Source: CAD feature listing. Evaluate the final solid. Frame: model axes, mm. A direction names the side the tool comes from. Round coordinates to 2 decimals unless told otherwise and drop trailing zeros. Loops run counter-clockwise (first coordinate to the right, second up) from the corner with the lowest first, then second, coordinate; pieces in that order, holes last. Notation, with made-up numbers: (71.5, -36) - (84.5, -36) arc R29 cw to (84.5, -1) - close; hole circle Ø4 at (-8, -39.75). An arc over 180 degrees is marked (long way). Write item = value, one per line. Start each with the question number.
from build123d import *

# Parameters (mm, degrees)
SKETCH1_R           = 5
BOSS_EXTRUDE1_DEPTH = 50
FILLET2_R           = 10
SKETCH2_R           = 12.5
CUT_EXTRUDE2_DEPTH  = 10


with BuildPart() as part:
    # Sketch1 → Boss-Extrude1 (new body)
    with BuildSketch(Plane.XY):
        with BuildLine():
            Line((0, 0), (0, 60))
            ThreePointArc((0, 60), (-20, 100), (0, 140))
            Line((0, 140), (0, 190))
            Line((0, 190), (-13.790104149, 190))
            Line((-13.790104149, 190), (-88.632697771, -15.62833599))
            Line((-88.632697771, -15.62833599), (0, 0))
        make_face()
        with Locations((-68.632697771, -1.947530257)):
            Circle(SKETCH1_R, mode=Mode.SUBTRACT)
        with Locations((-34.164426416, 4.130155961)):
            Circle(SKETCH1_R, mode=Mode.SUBTRACT)
    extrude(amount=BOSS_EXTRUDE1_DEPTH)

    # Fillet2
    # the kernel refuses this fillet: 10 mm, written as the material it takes off along each edge
    with BuildSketch(Plane(origin=(0, 0, -20.977490779), x_dir=(0, 1, 0), z_dir=(0, 0, 1))) as fillet2_piece_1:
        with BuildLine():
            CenterArc((FILLET2_R * 0.839099631177, FILLET2_R), FILLET2_R, 190, 80)
            Line((-FILLET2_R * 0.145708121835, FILLET2_R * 0.826351822333), (0, 0))
            Line((0, 0), (FILLET2_R * 0.839099631177, 0))
        make_face()
    extrude(amount=91.954981559, mode=Mode.SUBTRACT)
    with BuildSketch(Plane(origin=(-88.632697771, -15.62833599, -43.301270189), x_dir=(0.34202014332567615, 0.9396926207859058, 0), z_dir=(0, 0, 1))) as fillet2_piece_2:
        with BuildLine():
            CenterArc((FILLET2_R * 1.73205080757, -FILLET2_R), FILLET2_R, 90, 120)
            Line((FILLET2_R * 0.866025403784, -FILLET2_R * 1.5), (0, 0))
            Line((0, 0), (FILLET2_R * 1.73205080757, 0))
        make_face()
    extrude(amount=136.602540378, mode=Mode.SUBTRACT)
    with BuildSketch(Plane(origin=(-13.790104149, 190, -17.505188455), x_dir=(1, 0, 0), z_dir=(0, 0, 1))) as fillet2_piece_3:
        with BuildLine():
            CenterArc((FILLET2_R * 0.70020753821, -FILLET2_R), FILLET2_R, 90, 70)
            Line((-FILLET2_R * 0.239485082576, -FILLET2_R * 0.657979856674), (0, 0))
            Line((0, 0), (FILLET2_R * 0.70020753821, 0))
        make_face()
    extrude(amount=85.01037691, mode=Mode.SUBTRACT)
    with BuildSketch(Plane(origin=(0, 190, -25), x_dir=(0, -1, 0), z_dir=(0, 0, 1))) as fillet2_piece_4:
        with BuildLine():
            CenterArc((FILLET2_R, -FILLET2_R), FILLET2_R, 90, 90)
            Line((0, -FILLET2_R), (0, 0))
            Line((0, 0), (FILLET2_R, 0))
        make_face()
    extrude(amount=100, mode=Mode.SUBTRACT)

    # Sketch2 → Cut-Extrude2 (cut, symmetric)
    with BuildSketch(Plane.XY.offset(25)):
        with Locations((-68.632697771, -1.947530257)):
            Circle(SKETCH2_R)
    extrude(amount=CUT_EXTRUDE2_DEPTH, both=True, mode=Mode.SUBTRACT)


solid = part.part
(1) Cut plane A-A (x = -37). Output: boundary loops of the cut face in (y, z), and give its area (3 significant figures).
(2) Access query for faces 5 (the face through (-69.87, 10.49, 25.14)), 6 (the face through (-2, 186, 25)). Directions: +Z, -Z, +X, -X, +Y, -Y. A direction counts if a zero-diameter tool reaches every point of the face in a straight line with its end or side. Return the directions, or none.
(3) Cut plane C-C (z = 24.5). Output: boundary loops of the cut face in (x, y).
(4) Cut plane D-D (y = 40.5). Output: boundary loops of the cut face in (x, z).
(5) Cut plane B-B (z = 41). Output: boundary loops of the cut face in (x, y).
(6) Pin query (flat end, axial travel): P1, Ø4, axis at x = -52, z = 14, coming from the -Y side; P2, Ø8, axis at x = -66.5, z = 18.5, coming from the -Y side; P3, Ø12, axis at y = 119, z = 22.5, coming from the -X side; P4, Ø6, axis at x = -68.63, y = -1.95, coming from the +Z side. Return the tip coordinate at first contact, or that it passes through.
(7) Mould query, pull axis X, two halves, no side actions, for faces 1 (the face through (-69, 4, 35)), 2 (the face through (0, 160, 25)), 3 (the face through (-69, 4, 15)), 4 (the face through (-33, 67, 50)). Classes: +X half, -X half, draft (parallel to the pull), parting line (faces both ways), or undercut.
(8) Material intervals for line 1 along X through (y, z) = (53, 26.5); line 2 along X through (y, z) = (0.5, 37); line 3 along X through (y, z) = (25, 41.5), sorted ascending. Write a range as from..to.
Solution:
q1.outline = (-6.52, 0) - (0.01, 0) - (0.01, 50) - (-6.52, 50) - close; (8.25, 0) - (126.23, 0) - (126.23, 50) - (8.25, 50) - close
q1.area = 6,230 mm^2
q2.face_5 = none
q2.face_6 = +Z, -Z, +X, +Y
q3.outline = (-82.71, 0.65) arc R10 ccw to (-75.18, -12.6) arc R12.5 cw (long way) to (-59.51, -10.49) - (-8.26, -1.46) arc R10 ccw to (0, 8.39) - (0, 60) arc R50 cw to (0, 140) - (0, 180) arc R10 ccw to (-8.39, 189.87) arc R10 ccw to (-16.18, 183.42) - close; hole circle Ø10 at (-34.16, 4.13)
q4.outline = (-68.2, 0) - (0, 0) - (0, 50) - (-68.2, 50) - close
q5.outline = (-82.71, 0.65) arc R10 ccw to (-71.58, -12.62) - (-8.26, -1.46) arc R10 ccw to (0, 8.39) - (0, 60) arc R50 cw to (0, 140) - (0, 180) arc R10 ccw to (-8.39, 189.87) arc R10 ccw to (-16.18, 183.42) - close; hole circle Ø10 at (-68.63, -1.95); hole circle Ø10 at (-34.16, 4.13)
q6.P1 = -9.52
q6.P2 = -12.07
q6.P3 = -41.82
q6.P4 = through
q7.face_1 = undercut
q7.face_2 = +X half
q7.face_3 = undercut
q7.face_4 = draft
q8.line_1 = -63.65..0
q8.line_2 = -82.76..-72.99, -64.27..-37.6, -30.73..-3.86
q8.line_3 = -73.85..0
